from build123d import *

# Parameters (mm, degrees)
SKETCH_1_W      = 3
SKETCH_1_H      = 10
SKETCH_1_H_2    = 5
EXTRUDE_1_DEPTH = 3


with BuildPart() as part:
    # 草图1 → 凸台-拉伸1 (new body)
    with BuildSketch(Plane(origin=(0, 0, 0), x_dir=(1, 0, 0), z_dir=(0, 1, 0))):
        Polygon((0, -45), (0, -55), (10.5, -55), (10.5, -45), (10.5, -30), (10.5, -25), (10.5, -22), (0, -22), (0, -25), (0, -30), align=None)
        with Locations((12, -50)):
            Rectangle(SKETCH_1_W, SKETCH_1_H)
        with Locations((-1.5, -50)):
            Rectangle(SKETCH_1_W, SKETCH_1_H)
        with Locations((-1.5, -27.5)):
            Rectangle(SKETCH_1_W, SKETCH_1_H_2)
        with Locations((12, -27.5)):
            Rectangle(SKETCH_1_W, SKETCH_1_H_2)
    extrude(amount=EXTRUDE_1_DEPTH)


solid = part.part
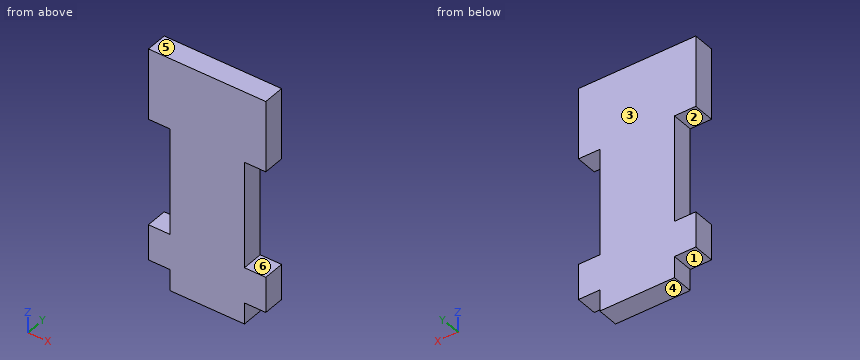
Geometry: final body of the model. Coordinates: model frame, mm. Face numbers are marked on the shaded views. A direction names the side the tool comes from. Give positions to 0.01 mm unless a question says otherwise; leave off trailing zeros. Write each loop counter-clockwise with the first axis right and the second up, starting at its lowest first coordinate (ties: lowest second). Pieces come first, ordered by that corner, then holes. Notation, with made-up numbers: (-5.75, 45.5) -> (19.25, 45.5) arc R24 ccw to (19.25, 83.5) -> close; hole circle Ø3 at (35.5, 6). An arc over 180 degrees is marked (long way). Answer in a Markdown table with one row per item.
(1) Ray query, line 1 along Z through (x, y) = (-1.5, 1.4); line 2 along X through (y, z) = (1.2, 33.5). Return the intervals inside material, ascending. Write a range as [from, to].
Answers below:
| item | result |
|---|---|
| line 1 | [25, 30], [45, 55] |
| line 2 | [0, 10.5] |
(2) Set-up query: the marked faces 1, 2 and 3. Return all of +Z, -Z, +X, -X, +Y, -Y with unobstructed straight access to the full face (end or side cutting, diameter ignored); none if empty.
Answers below:
| item | result |
|---|---|
| face 1 | -Z, -X, +Y, -Y |
| face 2 | -X, +Y, -Y |
| face 3 | +Z, -Z, +X, -X, +Y |
(3) Draft query along Z for the marked faces 4, 5 and 6. Return one class per face: +Z half, -Z half, draft (parallel to the pull), parting line (faces both ways), or undercut.
Answers below:
| item | result |
|---|---|
| face 4 | -Z half |
| face 5 | +Z half |
| face 6 | undercut |
(4) Section query A-A on x = 11. Return loops of the section in (y, z), then the cut area to 3 significant figures.
Answers below:
| item | result |
|---|---|
| outline | (0, 25) -> (3, 25) -> (3, 30) -> (0, 30) -> close; (0, 45) -> (3, 45) -> (3, 55) -> (0, 55) -> close |
| area | 45.0 mm^2 |
(5) Section query C-C on z = 34. Return loops of the section in (x, y).
Answers below:
| item | result |
|---|---|
| outline | (0, 0) -> (10.5, 0) -> (10.5, 3) -> (0, 3) -> close |
(6) Section query B-B on y = 0.55. Return loops of the section in (x, z).
Answers below:
| item | result |
|---|---|
| outline | (-3, 25) -> (0, 25) -> (0, 22) -> (10.5, 22) -> (10.5, 25) -> (13.5, 25) -> (13.5, 30) -> (10.5, 30) -> (10.5, 45) -> (13.5, 45) -> (13.5, 55) -> (-3, 55) -> (-3, 45) -> (0, 45) -> (0, 30) -> (-3, 30) -> close |
(7) Pin query (flat end, axial travel): pin 1 (0.9 mm diameter, centred on y = 2, z = 23.5, fed in from +X); pin 2 (1.5 mm diameter, centred on x = 12.5, y = 1.5, fed in from -Z); pin 3 (1.5 mm diameter, centred on y = 2, z = 24, fed in from -X). Return the tip coordinate at first contact, or that it passes through.
Answers below:
| item | result |
|---|---|
| pin 1 | x = 10.5 |
| pin 2 | z = 25 |
| pin 3 | x = 0 |
